Autodesk Fusion 360 part; units mm, degrees
sketch "Sketch1" plane through (0, 0, 0) normal (0, 0, 1) x (1, 0, 0)
  line L0 (-37.5, 0) -> (-37.5, 37.5)
  line L1 (-37.5, 37.5) -> (37.5, 37.5)
  line L2 (37.5, 37.5) -> (37.5, 0)
  arc A0 (-37.5, 0) -> (37.5, 0) centre (0, 0) ccw
  dimension "d1" = 75
  dimension "d2" = 75
extrude "Extrude1" add sketch "Sketch1" along normal blind 35
sketch "Sketch2" plane through (0, 37.5, 0) normal (0, 1, 0) x (-1, 0, 0)
  line L0 (-37.5, 0) -> (37.5, 0)
  line L1 (37.5, 0) -> (37.5, 35)
  line L2 (37.5, 35) -> (-37.5, 35)
  line L3 (-37.5, 35) -> (-37.5, 0)
  line L4 (37.5, 65) -> (-37.5, 65)
  line L5 (-37.5, 65) -> (-37.5, 25)
  line L6 (-37.5, 25) -> (37.5, 25)
  line L7 (37.5, 25) -> (37.5, 65)
  line L8 (37.5, 65) -> (-37.5, 25) construction
  line L9 (-37.5, 65) -> (37.5, 25) construction
  point P0 (0, 45)
  dimension "d6" = 75
  dimension "d7" = 40
extrude "Extrude2" add sketch "Sketch2" against normal blind 85 contours L2 L4 L5 L7
sketch "Sketch3" plane through (0, 0, 0) normal (0, 1, 0) x (1, 0, 0)
  circle A0 centre (0, -50) radius 8.5
  point P0 (0, -50)
  dimension "d12" = 17
extrude "Extrude3" add sketch "Sketch3" against normal blind 107.5
sketch "Sketch4" plane through (0, -107.5, 0) normal (0, -1, 0) x (1, 0, 0)
  circle A0 centre (0, 50) radius 8.5
  circle A1 centre (0, 50) radius 7.5
  dimension "d15" = 15
extrude "Extrude4" cut sketch "Sketch4" against normal blind 40
sketch "Sketch5" plane through (0, 0, 0) normal (0, 0, -1) x (-1, 0, 0)
  line L0 (37.5, 0) -> (37.5, 37.5)
  line L1 (37.5, 37.5) -> (-37.5, 37.5)
  line L2 (-37.5, 37.5) -> (-37.5, 0)
  arc A0 (-37.5, 0) -> (37.5, 0) centre (0, 0) ccw
  line L3 (0, 37.5) -> (0, 27.5)
  line L4 (-37.5, 0) -> (-27.5, 0)
  line L5 (37.5, 0) -> (27.5, 0)
  line L6 (0, -37.5) -> (0, -27.5)
  dimension "d18" = 10
  dimension "d19" = 10
  dimension "d20" = 10
  dimension "d21" = 10
extrude "Extrude6" cut 1 faces at (-12.5, 25, 0) along direction (0, 0, 1) blind 20
sketch "Sketch6" plane through (0, -107.5, 0) normal (0, -1, 0) x (1, 0, 0)
  circle A0 centre (0, 50) radius 7.5
  circle A1 centre (0, 50) radius 7.5
extrude "Extrude7" add sketch "Sketch6" along normal blind 10
sketch "Sketch7" plane through (0, -117.5, 0) normal (0, -1, 0) x (1, 0, 0)
  circle A0 centre (0, 50) radius 7.5
  circle A1 centre (0, 50) radius 2
  dimension "d33" = 4
extrude "Extrude8" add sketch "Sketch7" along normal blind 14.509 contours A1
sketch "Sketch8" plane through (0, 0, 65) normal (0, 0, 1) x (1, 0, 0)
  line L0 (37.5, 37.5) -> (-37.5, 37.5)
  line L1 (-37.5, 37.5) -> (-37.5, -47.5)
  line L2 (-37.5, -47.5) -> (37.5, -47.5)
  line L3 (37.5, -47.5) -> (37.5, 37.5)
  line L4 (0, 37.5) -> (0, 27.5)
  line L5 (-37.5, 0) -> (-27.5, 0)
  line L6 (0, -37.5) -> (0, -27.5)
  line L7 (37.5, 0) -> (27.5, 0)
  dimension "d36" = 10
  dimension "d38" = 360
hole "Hole2" at (0, 27.5, 65) at (27.5, 0, 65) at (-27.5, 0, 65) at (0, -27.5, 65) direction (0, 0, -1) diameter 3.332 end through all counterbore diameter 8 counterbore depth 1
Geometry check sheet. Reference: the model listing, model coordinates, mm. A direction names the side the tool comes from. Round coordinates to 2 decimals unless told otherwise and drop trailing zeros. Order: outer loops, then holes, each group sorted by start corner. A loop starts at its lowest first (then second) coordinate and runs counter-clockwise, first axis right, second up. Notation, with made-up numbers: M 71,59.25 L 90,59.25 A15 ccw 90,85.25 Z; hole C -17,56 d3. An arc over 180 degrees is marked long. Answer in a Markdown table with one row per item. Add a question column.
Item 1: Sectioned sample at C-C, the plane x = 0. State how many separate pieces and enclosed holes the cut face has, plus the area to 3 significant figures.
Item 2: Set-up check for faces 1 (the face through (-37.5, -6, 47)), 2 (the face through (0, -67.5, 42)), 3 (the face through (0.82, -37.49, 27.4)), 4 (the face through (27, -2, 64)): record each of +Z, -Z, +X, -X, +Y, -Y from which the full face is reachable in a straight line by a thin tool's end or side.
Item 3: Draft check along Y on faces 5 (the face through (-1.84, -57.36, 58.3)), 6 (the face through (-31.466, 0.521, 64.493)), 7 (the face through (0, -132.009, 50)). Enter one of: released by +Y, released by -Y, zero draft, split by the parting line, or undercut.
Item 4: Depth check by flat-ended pin: pin 1 Ø12 at (x, z) = (5, 40.5) entering from -Y; pin 2 Ø3 at (x, y) = (-6, -78) entering from -Z; pin 3 Ø5 at (x, y) = (27.5, 0) entering from +Z; pin 4 Ø3 at (x, y) = (0, -27.5) entering from +Z. Enter the tip coordinate at first touch or a pass-through.
Item 5: Sectioned sample at B-B, the plane y = -27.5. Enter the section's corners in (x, z), plus the area to 3 significant figures.
Item 6: Material ranges on L1, parallel to X at y = 0, z = 55.5; L2, parallel to Y at x = 0, z = 44; L3, parallel to Y at x = -27.5, z = 36, recorded low to high. Write a range as [from, to].
Item 7: Sectioned sample at D-D, the plane x = -27.5. Enter the section's corners in (y, z), plus the area to 3 significant figures.
Item 8: Sectioned sample at A-A, the plane z = 30. Enter the section's corners in (x, y).
Filled in:
| question | item | result |
|---|---|---|
| 1 | separate pieces | 3 |
| 1 | enclosed holes | 0 |
| 1 | area | 4,510 mm² |
| 2 | face 1 | +Z, -Z, -X, +Y, -Y |
| 2 | face 2 | -Y |
| 2 | face 3 | -Z, -Y |
| 2 | face 4 | +Z |
| 3 | face 5 | zero draft |
| 3 | face 6 | undercut |
| 3 | face 7 | released by -Y |
| 4 | pin 1 | stops at y = -117.5 |
| 4 | pin 2 | stops at z = 44 |
| 4 | pin 3 | stops at z = 64 |
| 4 | pin 4 | passes through |
| 5 | outline | M -37.5,35 L -25.5,35 L -25.5,20 L -1.67,20 L -1.67,64 L -4,64 L -4,65 L -37.5,65 Z; M 1.67,20 L 25.5,20 L 25.5,35 L 37.5,35 L 37.5,65 L 4,65 L 4,64 L 1.67,64 Z |
| 5 | area | 2,860 mm² |
| 6 | L1 | x = [-37.5, -29.17], [-25.83, 25.83], [29.17, 37.5] |
| 6 | L2 | y = [-117.5, -29.17], [-25.83, 25.83], [29.17, 37.5] |
| 6 | L3 | y = [-47.5, -1.67], [1.67, 37.5] |
| 7 | outline | M -47.5,35 L -25.5,35 L -25.5,20 L -1.67,20 L -1.67,64 L -4,64 L -4,65 L -47.5,65 Z; M 1.67,20 L 37.5,20 L 37.5,65 L 4,65 L 4,64 L 1.67,64 Z |
| 7 | area | 3,340 mm² |
| 8 | outline | M -37.5,0 A37.5 ccw 37.5,0 L 37.5,37.5 L -37.5,37.5 Z; hole C -27.5,0 d3.33; hole C 0,-27.5 d3.33; hole C 0,27.5 d3.33; hole C 27.5,0 d3.33 |
